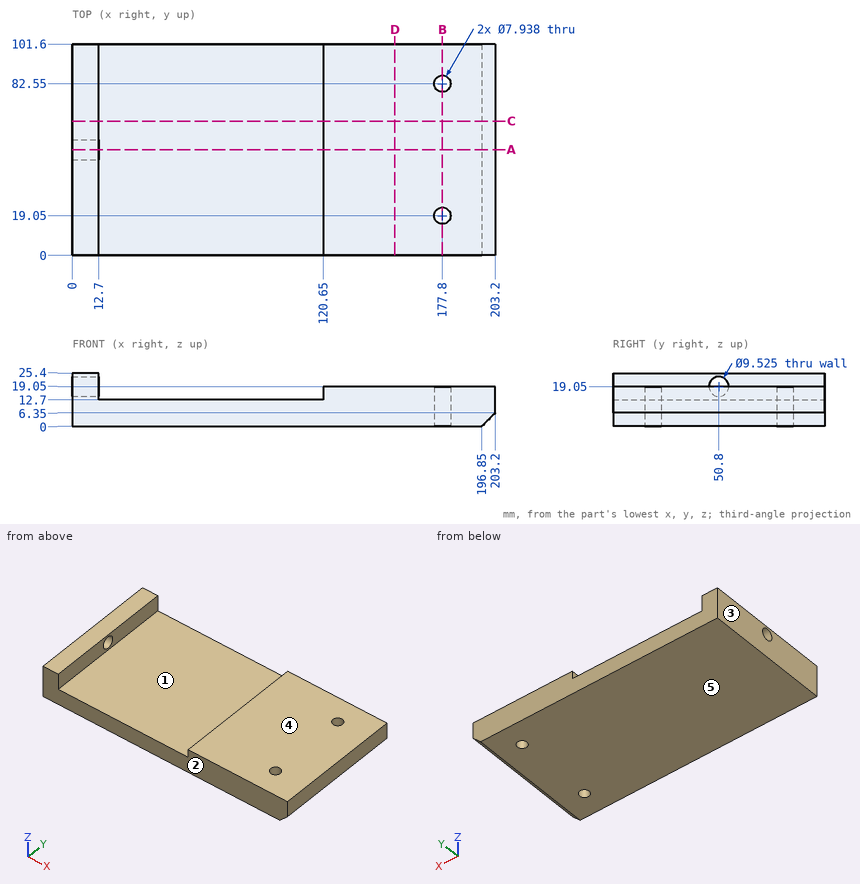
Geometry check sheet. Reference: drawing and pictorial views, mm from the part's lowest x, y, z. A direction names the side the tool comes from. Coordinates: 2 decimals unless noted, no trailing zeros. Loops run counter-clockwise (first coordinate to the right, second up) from the corner with the lowest first, then second, coordinate; pieces in that order, holes last. Notation, with made-up numbers: (65, 11) - (120, 11) arc R8 cw to (120, 21) - close; hole circle Ø1 at (86.25, 63.25). An arc over 180 degrees is marked (long way). Return JSON: item names as keys, results as strings.
1. Mould release check, pull along X, two halves, no side actions. Record for the marked faces 1, 2 and 3: +X half, -X half, draft (parallel to the pull), parting line (faces both ways), or undercut.
Established:
{"face 1": "undercut", "face 2": "draft", "face 3": "-X half"}
2. Section check A-A, the plane y = 50.8. Record the boundary of the cut face in (x, z), then the cut area to 4 significant figures.
Established:
{"outline": "(0, 0) - (196.85, 0) - (203.2, 6.35) - (203.2, 19.05) - (120.65, 19.05) - (120.65, 12.7) - (12.7, 12.7) - (12.7, 14.29) - (0, 14.29) - close; (0, 23.81) - (12.7, 23.81) - (12.7, 25.4) - (0, 25.4) - close", "area": "3,125 mm2"}
3. Tool access check on the marked faces 4 and 5. Record the directions out of +Z, -Z, +X, -X, +Y, -Y that give a thin tool (end or side, any length) a straight path to the whole face; none if there is none.
Established:
{"face 4": "+Z, +X, +Y, -Y", "face 5": "-Z, +X, -X, +Y, -Y"}
4. Section check D-D, the plane x = 155. Record the boundary of the cut face in (y, z).
Established:
{"outline": "(0, 0) - (101.6, 0) - (101.6, 19.05) - (0, 19.05) - close"}
5. Thickness scan on L1, parallel to Y at x = 177.8, z = 12.25; L2, parallel to Z at x = 10.25, y = 50.8; L3, parallel to Z at x = 34.5, y = 5. Record the ranges inside material, lowest first.
Established:
{"L1": "y = 0 to 15.08, 23.02 to 78.58, 86.52 to 101.6", "L2": "z = 0 to 14.29, 23.81 to 25.4", "L3": "z = 0 to 12.7"}
6. Section check B-B, the plane x = 177.8. Record the boundary of the cut face in (y, z).
Established:
{"outline": "(0, 0) - (15.08, 0) - (15.08, 19.05) - (0, 19.05) - close; (23.02, 0) - (78.58, 0) - (78.58, 19.05) - (23.02, 19.05) - close; (86.52, 0) - (101.6, 0) - (101.6, 19.05) - (86.52, 19.05) - close"}
7. Go/stop test with flat-tipped pins: pin 1 (7 mm diameter, centred on x = 177.8, y = 82.55, fed in from -Z); pin 2 (8 mm diameter, centred on x = 175.5, y = 55.5, fed in from +Z); pin 3 (8.5 mm diameter, centred on y = 50.8, z = 19.05, fed in from -X). Record where each tip stops, or that it passes through.
Established:
{"pin 1": "passes through", "pin 2": "stops at z = 19.05", "pin 3": "stops at x = 120.65"}
8. Section check C-C, the plane y = 64.5. Record the boundary of the cut face in (x, z).
Established:
{"outline": "(0, 0) - (196.85, 0) - (203.2, 6.35) - (203.2, 19.05) - (120.65, 19.05) - (120.65, 12.7) - (12.7, 12.7) - (12.7, 25.4) - (0, 25.4) - close"}
